```python
from build123d import *

# Parameters (mm, degrees)
EXTRUDE_1_DEPTH     = 8
SKETCH_2_R          = 1.6
CUT_EXTRUDE_1_DEPTH = 10


with BuildPart() as part:
    # Эскиз1 → Бобышка-Вытянуть1 (new body)
    with BuildSketch(Plane(origin=(0, 0, 0), x_dir=(1, 0, 0), z_dir=(0, 1, 0))):
        with BuildLine():
            Line((120.67483279, 57.76097026), (125.67483279, 57.76097026))
            add(Edge.make_bspline(
                [(25.67483279, -2.23902974), (121.28759337, -7.643443061), (125.67483279, 57.76097026)],
                knots=[0, 0, 0, 1, 1, 1], degree=2))
            Line((25.67483279, -2.23902974), (-4.32516721, -2.23902974))
            Line((-4.32516721, -2.23902974), (-4.32516721, 2.76097026))
            Line((-4.32516721, 2.76097026), (25.67483279, 2.76097026))
            add(Edge.make_bspline(
                [(25.67483279, 2.76097026), (115.69323106, -1.985762605), (120.67483279, 57.76097026)],
                knots=[0, 0, 0, 1, 1, 1], degree=2))
        make_face()
    extrude(amount=EXTRUDE_1_DEPTH)

    # Эскиз2 → Вырез-Вытянуть1 (cut)
    with BuildSketch(Plane(origin=(0, 0, -2.76097026), x_dir=(-1, 0, 0), z_dir=(0, 0, -1))):
        with Locations((-22.01483279, 4)):
            Circle(SKETCH_2_R)
        with Locations((1.32516721, 4)):
            Circle(SKETCH_2_R)
    extrude(amount=-CUT_EXTRUDE_1_DEPTH, mode=Mode.SUBTRACT)


solid = part.part
```
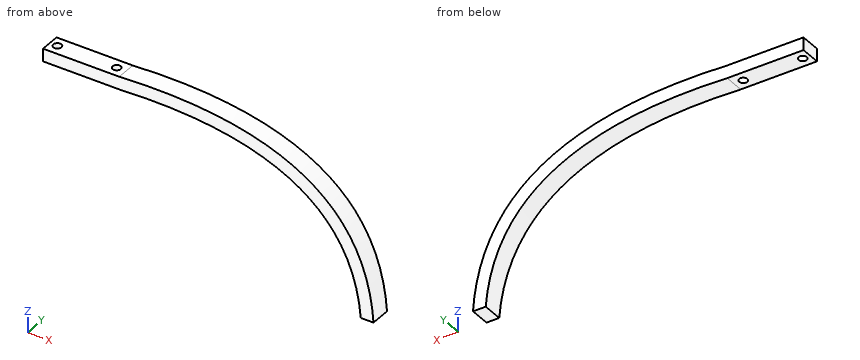
Can you work these out from the model? Positions are in its coordinate system, mm. Coordinates: 2 decimals unless noted, no trailing zeros. Answer as a JSON object with one key per item and string values.
1) If I drill on line 1 (Z direction, x = 14, y = 6.75); line 2 (X direction, y = 1.75, z = -42); line 3 (Z direction, x = 40, y = 1.75), over which ranges is the centre line in solid material (lowest first)?
Results:
{"line 1": "z = -2.76 to 2.24", "line 2": "x = 117.51 to 123.01", "line 3": "z = -2.42 to 2.65"}
2) For P1, Ø1, axis at y = 5.5, z = -11, coming from the -X side; P2, Ø4, axis at x = 4.5, y = 3, coming from the -Z side; P3, Ø2.5, axis at x = 9, y = 3, coming from the +Z side; P4, Ø8, axis at x = 82, z = -13.5, coming from the -Y side, each with a flat end and sliding along its axis, tell me the tip position at first contact or that it passes through.
Results:
{"P1": "stops at x = 87.13", "P2": "stops at z = -2.76", "P3": "stops at z = 2.24", "P4": "passes through"}
3) Imagine slicing it at A-A (y = 4). Count the separate pieces of the cut face and the enclosed holes in it, then the cut area to 3 significant figures.
Results:
{"separate pieces": "3", "enclosed holes": "0", "area": "797 mm^2"}
